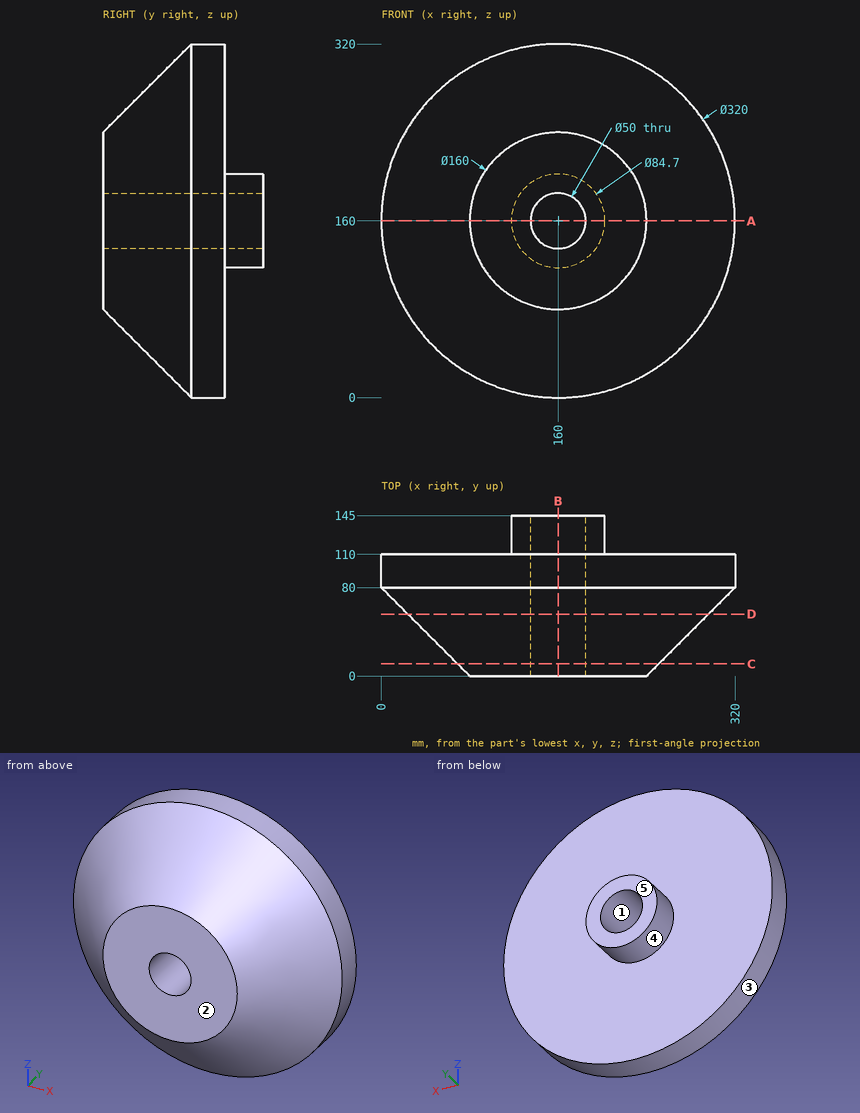
Input: dimensioned drawing with shaded views. Units: mm. Origin: part minimum x, y, z. A direction names the side the tool comes from. Coordinates: 2 decimals unless noted, no trailing zeros. Write each loop counter-clockwise with the first axis right and the second up, starting at its lowest first coordinate (ties: lowest second). Pieces come first, ordered by that corner, then holes. Notation, with made-up numbers: M 56.5,-9.5 L 79.5,-9.5 A26 cw 79.5,11.5 Z; hole C 29.25,-11.5 d1. An arc over 180 degrees is marked long. Use a Markdown table: item, result.
1) Section A-A, the plane z = 160. Output: boundary loops of the cut face in (x, y), then the cut area to 3 significant figures.
Conclusion:
| item | result |
|---|---|
| outline | M 0,80 L 80,0 L 135,0 L 135,145 L 117.65,145 L 117.65,110 L 0,110 Z; M 185,0 L 240,0 L 320,80 L 320,110 L 202.35,110 L 202.35,145 L 185,145 Z |
| area | 24,500 mm^2 |
2) Reachability of the marked faces 4 and 5 from +Z, -Z, +X, -X, +Y, -Y: full face, straight path, thin tool, end or side. Return the list, or none.
Conclusion:
| item | result |
|---|---|
| face 4 | +Y |
| face 5 | +Z, -Z, +X, -X, +Y |
3) Section B-B, the plane x = 160. Output: boundary loops of the cut face in (y, z).
Conclusion:
| item | result |
|---|---|
| outline | M 0,80 L 80,0 L 110,0 L 110,117.65 L 145,117.65 L 145,135 L 0,135 Z; M 0,185 L 145,185 L 145,202.35 L 110,202.35 L 110,320 L 80,320 L 0,240 Z |
4) First-contact query: pin 1 Ø4 at (x, z) = (97.5, 65) entering from +Y; pin 2 Ø12 at (x, y) = (253.5, 95.5) entering from -Z; pin 3 Ø10 at (y, z) = (34.5, 125.5) entering from +X. Flat tips, straight axial feed; report the tip coordinate or a pass-through.
Conclusion:
| item | result |
|---|---|
| pin 1 | stops at y = 110 |
| pin 2 | stops at z = 26.05 |
| pin 3 | stops at x = 274.62 |
5) Section D-D, the plane y = 56. Output: boundary loops of the cut face in (x, z), then the cut area to 3 significant figures.
Conclusion:
| item | result |
|---|---|
| outline | C 160,160 d272; hole C 160,160 d50 |
| area | 56,100 mm^2 |
6) Ray query, L1, parallel to Z at x = 160, y = 86.5; L2, parallel to Z at x = 162.5, y = 8; L3, parallel to X at y = 83.5, z = 137.5. Return the intervals inside material, ascending.
Conclusion:
| item | result |
|---|---|
| L1 | z = 0 to 135, 185 to 320 |
| L2 | z = 72.04 to 135.13, 184.87 to 247.96 |
| L3 | x = 1.59 to 149.1, 170.9 to 318.41 |
7) Section C-C, the plane y = 11. Output: boundary loops of the cut face in (x, z), then the cut area to 3 significant figures.
Conclusion:
| item | result |
|---|---|
| outline | C 160,160 d182; hole C 160,160 d50 |
| area | 24,100 mm^2 |
8) Mould query, pull axis X, two halves, no side actions, for the marked faces 1, 2 and 3. Classes: pulls with the +X half, pulls with the -X half, needs draft (parallel to the pull), parting line crosses it, or undercut.
Conclusion:
| item | result |
|---|---|
| face 1 | undercut |
| face 2 | needs draft |
| face 3 | parting line crosses it |
